Part model, mm, in its own coordinate system. Face numbers are marked on the shaded views. A direction names the side the tool comes from. Give positions to 0.01 mm unless a question says otherwise; leave off trailing zeros. Order: outer loops, then holes, each group sorted by start corner. A loop starts at its lowest first (then second) coordinate and runs counter-clockwise, first axis right, second up. Notation, with made-up numbers: M 43.25,-35 L 74.25,-35 A15 ccw 74.25,-6 Z; hole C 56.25,37.25 d10. An arc over 180 degrees is marked long. One line per question, with ' | ' between items.
```python
from build123d import *

# Parameters (mm, degrees)
SKETCH1_W          = 75
SKETCH1_H          = 6.35
BASE_EXTRUDE_DEPTH = 19.05
CUT_EXTRUDE1_DEPTH = 78.641644753
SKETCH3_R          = 2.38125
CUT_EXTRUDE2_DEPTH = 78.641644753


with BuildPart() as part:
    # Sketch1 → Base-Extrude (new body)
    with BuildSketch(Plane.XY):
        with Locations((37.5, 3.175)):
            Rectangle(SKETCH1_W, SKETCH1_H)
    extrude(amount=BASE_EXTRUDE_DEPTH)

    # Sketch2 → Cut-Extrude1 (cut, through all)
    with BuildSketch(Plane(origin=(0, 6.35, 0), x_dir=(-1, 0, 0), z_dir=(0, 1, 0))):
        with BuildLine():
            Line((-70.3645, 5.473421326), (-70.3645, 13.576578674))
            ThreePointArc((-70.3645, 13.576578674), (-59.125, 9.525), (-70.3645, 5.473421326))
        make_face()
    extrude(amount=-CUT_EXTRUDE1_DEPTH, mode=Mode.SUBTRACT)

    # Sketch3 → Cut-Extrude2 (cut, through all)
    with BuildSketch(Plane(origin=(0, 6.35, 0), x_dir=(-1, 0, 0), z_dir=(0, 1, 0))):
        with Locations((-9.525, 9.525)):
            Circle(SKETCH3_R)
    extrude(amount=-CUT_EXTRUDE2_DEPTH, mode=Mode.SUBTRACT)


solid = part.part
```
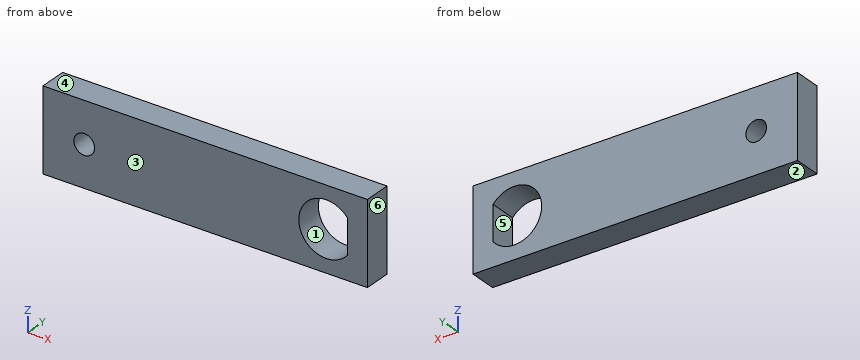
1. Slice it at B-B on z = 4.5. Give the cut face in (x, y).
Worked out:
outline: M 0,0 L 61.59,0 L 61.59,6.35 L 0,6.35 Z; M 69.36,0 L 75,0 L 75,6.35 L 69.36,6.35 Z
2. Tool access for the marked faces 5 and 6: list every direction of +Z, -Z, +X, -X, +Y, -Y with a clear straight run to the whole face (end or side of a thin tool).
Worked out:
face 5: +Y, -Y | face 6: +Z, -Z, +X, +Y, -Y
3. Slice it at A-A on z = 10.5. Give the cut face in (x, y), then the cut area to 3 significant figures.
Worked out:
outline: M 0,0 L 7.35,0 L 7.35,6.35 L 0,6.35 Z; M 11.7,0 L 59.2,0 L 59.2,6.35 L 11.7,6.35 Z; M 70.36,0 L 75,0 L 75,6.35 L 70.36,6.35 Z | area: 378 mm2
4. Mould opens along Z. For the marked faces 1, 2, 3 and 4 say: released by +Z, released by -Z, zero draft, split by the parting line, or undercut.
Worked out:
face 1: undercut | face 2: released by -Z | face 3: zero draft | face 4: released by +Z
5. Slice it at C-C on y = 5.25. Give the number of separate pieces and of enclosed holes in the cut face, then the cut area to 3 significant figures.
Worked out:
separate pieces: 1 | enclosed holes: 2 | area: 1,290 mm2
6. Probe L1, parallel to X at y = 2.5, z = 11; L2, parallel to Z at x = 7.5, y = 3.75; L3, parallel to X at y = 5.5, z = 9. List the from-to ranges inside material, lowest first. Write a range as from..to.
Worked out:
L1: x = 0..7.66, 11.39..59.3, 70.36..75 | L2: z = 0..8.27, 10.78..19.05 | L3: x = 0..7.2, 11.85..59.15, 70.36..75
